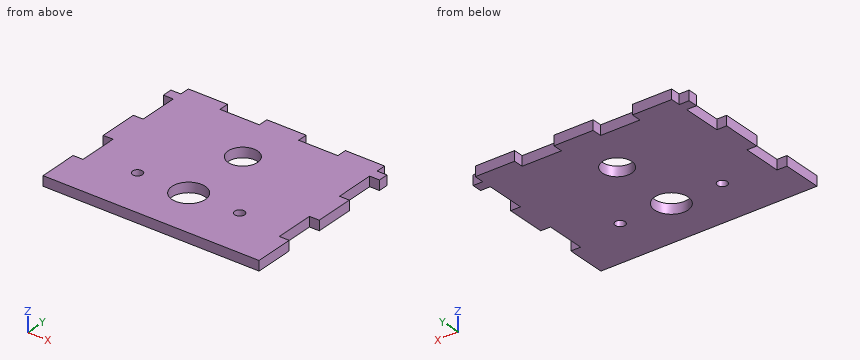
```python
from build123d import *

# Parameters (mm, degrees)
SKETCH_1_W                       = 100
SKETCH_1_H                       = 85
SKETCH_1_R                       = 8.5
SKETCH_1_R_2                     = 2.5
SKETCH_1_R_3                     = 7.5
EXTRUDE_1_DEPTH                  = 5
SKETCH_2_W                       = 5
SKETCH_2_H                       = 20
EXTRUDE_2_DEPTH                  = 5
PATTERN_LINEAR_1_COUNT           = 2
PATTERN_LINEAR_1_PITCH           = 40
PATTERN_LINEAR_1_COPY_1_SKETCH_W = 5
PATTERN_LINEAR_1_COPY_1_SKETCH_H = 20
PATTERN_LINEAR_1_COPY_1_DEPTH    = 5
SKETCH_3_W                       = 20
SKETCH_3_H                       = 5
EXTRUDE_3_DEPTH                  = 5
PATTERN_LINEAR_2_COUNT           = 2
PATTERN_LINEAR_2_PITCH           = 40
PATTERN_LINEAR_3_COUNT           = 2
PATTERN_LINEAR_3_PITCH           = 40
SKETCH_5_W                       = 5
SKETCH_5_H                       = 5
EXTRUDE_4_DEPTH                  = 5


with BuildPart() as part:
    # 스케치1 → 보스-돌출1 (new body)
    with BuildSketch(Plane.XY):
        Rectangle(SKETCH_1_W, SKETCH_1_H)
        with Locations((0, -17.5)):
            Circle(SKETCH_1_R, mode=Mode.SUBTRACT)
        with Locations((-26, -17.5)):
            Circle(SKETCH_1_R_2, mode=Mode.SUBTRACT)
        with Locations((26, -17.5)):
            Circle(SKETCH_1_R_2, mode=Mode.SUBTRACT)
        with Locations((0, 18.5)):
            Circle(SKETCH_1_R_3, mode=Mode.SUBTRACT)
    extrude(amount=EXTRUDE_1_DEPTH)

    # 스케치2 → 보스-돌출2 (add)
    with BuildSketch(Plane.XY.offset(5)):
        with Locations((52.5, -32.5)):
            Rectangle(SKETCH_2_W, SKETCH_2_H)
    extrude_2 = extrude(amount=-EXTRUDE_2_DEPTH)

    # 대칭 복사1: 보스-돌출2 across plane
    add(extrude_2.mirror(Plane(origin=(0, 0, 0), x_dir=(0, 0, 1), z_dir=(1, 0, 0))))

    # 선형 패턴1: 보스-돌출2 ×2
    with Locations(*[(0, i * PATTERN_LINEAR_1_PITCH, 0) for i in range(1, PATTERN_LINEAR_1_COUNT)]):
        add(extrude_2)

    # 선형 패턴1 copy 1 sketch → 선형 패턴1 copy 1 (add)
    with BuildSketch(Plane(origin=(0, 40, 5), x_dir=(-1, 0, 0), z_dir=(0, 0, 1))):
        with Locations((52.5, 32.5)):
            Rectangle(PATTERN_LINEAR_1_COPY_1_SKETCH_W, PATTERN_LINEAR_1_COPY_1_SKETCH_H)
    extrude(amount=-PATTERN_LINEAR_1_COPY_1_DEPTH)

    # 스케치3 → 보스-돌출3 (add)
    with BuildSketch(Plane.XY.offset(5)):
        with Locations((0, 45)):
            Rectangle(SKETCH_3_W, SKETCH_3_H)
    extrude_3 = extrude(amount=-EXTRUDE_3_DEPTH)

    # 선형 패턴2: 보스-돌출3 ×2
    with Locations(*[(i * PATTERN_LINEAR_2_PITCH, 0, 0) for i in range(1, PATTERN_LINEAR_2_COUNT)]):
        add(extrude_3)

    # 선형 패턴3: 보스-돌출3 ×2
    with Locations(*[(-i * PATTERN_LINEAR_3_PITCH, 0, 0) for i in range(1, PATTERN_LINEAR_3_COUNT)]):
        add(extrude_3)

    # 스케치5 → 보스-돌출4 (add)
    with BuildSketch(Plane.XY.offset(5)):
        with Locations((52.5, 40)):
            Rectangle(SKETCH_5_W, SKETCH_5_H)
    extrude_4 = extrude(amount=-EXTRUDE_4_DEPTH)

    # 대칭 복사2: 보스-돌출4 across plane
    add(extrude_4.mirror(Plane(origin=(0, 0, 0), x_dir=(0, 0, 1), z_dir=(1, 0, 0))))


solid = part.part
```
Geometry check sheet. Reference: the model listing, model coordinates, mm. Give positions to 0.01 mm unless a question says otherwise; leave off trailing zeros. Loops run counter-clockwise (first coordinate to the right, second up) from the corner with the lowest first, then second, coordinate; pieces in that order, holes last. Notation, with made-up numbers: (89, 19) - (144, 19) arc R33 cw to (144, 54) - close; hole circle Ø2 at (-29.75, 81). An arc over 180 degrees is marked (long way). Use CSV: the item, a comma, the result in double quotes. Start each with the question number.
Q1. Section check C-C, the plane x = -26. Record the cut outline in (y, z), and give its area (3 significant figures).
Q2. Section check B-B, the plane y = -17.5. Record the cut outline in (x, z).
Q3. Section check A-A, the plane x = 0. Record the cut outline in (y, z), and give its area (3 significant figures).
Q4. Scan lines: probe 1 along Y at (x, z) = (0, 3.65); probe 2 along Y at (x, z) = (18, 4.65); probe 3 along Y at (x, z) = (26, 3.2). Record each from-to range of solid material in increasing order. Write a range as from..to.
Q5. Go/stop test with flat-tipped pins: pin 1 Ø1.5 at (y, z) = (44, 3) entering from -X; pin 2 Ø1.5 at (y, z) = (45.5, 3) entering from +X; pin 3 Ø1.5 at (x, z) = (51.5, 2.5) entering from +Y; pin 4 Ø19.5 at (x, y) = (0, -17.5) entering from -Z. Record where each tip stops, or that it passes through.
Q6. Section check D-D, the plane y = 21.5. Record the cut outline in (x, z).
Findings below:
1,outline,"(-42.5, 0) - (-20, 0) - (-20, 5) - (-42.5, 5) - close; (-15, 0) - (42.5, 0) - (42.5, 5) - (-15, 5) - close"
1,area,"400 mm^2"
2,outline,"(-50, 0) - (-28.5, 0) - (-28.5, 5) - (-50, 5) - close; (-23.5, 0) - (-8.5, 0) - (-8.5, 5) - (-23.5, 5) - close; (8.5, 0) - (23.5, 0) - (23.5, 5) - (8.5, 5) - close; (28.5, 0) - (50, 0) - (50, 5) - (28.5, 5) - close"
3,outline,"(-42.5, 0) - (-26, 0) - (-26, 5) - (-42.5, 5) - close; (-9, 0) - (11, 0) - (11, 5) - (-9, 5) - close; (26, 0) - (47.5, 0) - (47.5, 5) - (26, 5) - close"
3,area,"290 mm^2"
4,probe 1,"y = -42.5..-26, -9..11, 26..47.5"
4,probe 2,"y = -42.5..42.5"
4,probe 3,"y = -42.5..-20, -15..42.5"
5,pin 1,"stops at x = -50"
5,pin 2,"stops at x = 50"
5,pin 3,"stops at y = 42.5"
5,pin 4,"stops at z = 0"
6,outline,"(-50, 0) - (-6.87, 0) - (-6.87, 5) - (-50, 5) - close; (6.87, 0) - (50, 0) - (50, 5) - (6.87, 5) - close"
